Geometry check sheet. Reference: the model listing, model coordinates, mm. Round coordinates to 2 decimals unless told otherwise and drop trailing zeros. Write each loop counter-clockwise with the first axis right and the second up, starting at its lowest first coordinate (ties: lowest second). Pieces come first, ordered by that corner, then holes. Notation, with made-up numbers: M -1,70.25 L 22,70.25 A14 cw 22,79.25 Z; hole C 39,76 d11. An arc over 180 degrees is marked long. One line per item, written item: value. Start each with the question number.
1. Depth check by flat-ended pin: P1, Ø8, axis at x = 7, y = 14, coming from the -Z side; P2, Ø8, axis at y = 11.5, z = 778.5, coming from the +X side (3 decimals); P3, Ø5, axis at y = 6.5, z = 552.5, coming from the +X side; P4, Ø5, axis at x = 12, y = 7.5, coming from the -Z side. Enter the tip coordinate at first touch or a pass-through.
2. Scan lines: probe 1 along X at (y, z) = (18.5, 670.5) (3 decimals); probe 2 along Z at (x, y) = (1.75, 22.25). Record each from-to range of solid material in increasing order. Write a range as [from, to].
3. Section check C-C (y = 10.5). Record the boundary of the cut face in (x, z) (3 decimals).
4. Section check A-A (z = 879.5). Record the boundary of the cut face in (x, y) (3 decimals), and give its area (3 significant figures).
5. Section check B-B (x = 14). Record the boundary of the cut face in (y, z) (3 decimals).
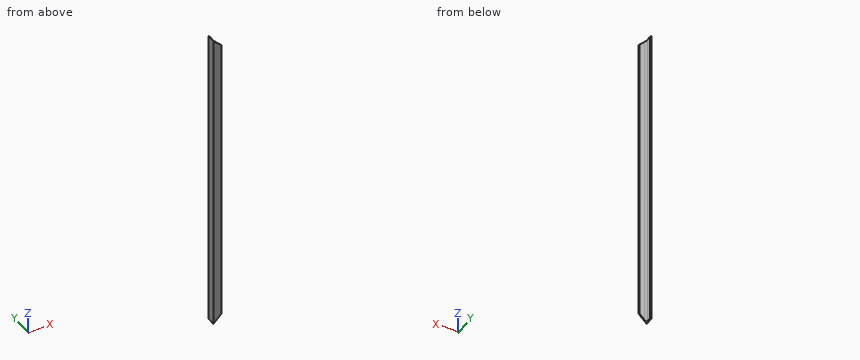
Autodesk Inventor part; units mm, degrees
ref_plane "Start Plane" through (0, 0, 0) normal (0, 0, 1) x (1, 0, 0)
ref_plane "End Plane" through (0, 0, 1000) normal (0, 0, 1) x (1, 0, 0)
ref_plane "Work Plane30" through (-0.0013, 12.7013, 0) normal (0.7071, -0.0001, -0.7071) x (-0.7071, 0.0002, -0.7071)
ref_plane "Start Plane" through (0, 0, 0) normal (0, 0, 1) x (1, 0, 0)
ref_plane "End Plane" through (0, 0, 1000) normal (0, 0, 1) x (1, 0, 0)
sketch "Sketch" plane through (0, 0, 0) normal (0, 0, 1) x (1, 0, 0)
  line L0 (25.4, 0) -> (0, 0)
  line L1 (0, 0) -> (0, 25.4)
  line L2 (0, 25.4) -> (1.651, 25.4)
  line L3 (3.175, 23.876) -> (3.175, 6.477)
  line L4 (6.477, 3.175) -> (23.876, 3.175)
  line L5 (25.4, 1.651) -> (25.4, 0)
  line L6 (0, -11.0414) -> (0, 31.5385) construction
  line L7 (-11.0414, 0) -> (31.5385, 0) construction
  arc A0 (3.175, 6.477) -> (6.477, 3.175) centre (6.477, 6.477) ccw
  arc A1 (3.175, 23.876) -> (1.651, 25.4) centre (1.651, 23.876) ccw
  arc A2 (25.4, 1.651) -> (23.876, 3.175) centre (23.876, 1.651) ccw
  line L8 (0, 40.0545) -> (0, -19.5574) construction
  line L9 (-19.5574, 0) -> (40.0545, 0) construction
  point P0 (3.175, 25.4)
  point P1 (3.175, 3.175)
  point P2 (25.4, 3.175)
  dimension "d0" = 25.4
  dimension "d1" = 25.4
  dimension "d2" = 3.175
  dimension "d3" = 3.175
  dimension "d10" = 0
  dimension "d11" = 0
  dimension "d14" = 3.302
  dimension "d15" = 1.524
extrude "Body" add sketch "Sketch" along normal up to surface (1000 mm away) from surface at 0
sketch "Sketch3" plane through (0, 0, 0) normal (0, 0, 1) x (1, 0, 0)
  line L0 (0, 0) -> (10, 0)
ref_plane "Work Plane3" through (0, 0, 0) normal (0, -1, 0) x (1, 0, 0)
ref_plane "Work Plane30" through (-0.0013, 12.7013, 0) normal (0.7071, -0.0001, -0.7071) x (-0.7071, 0.0002, -0.7071)
split "Split3" plane through (-0.0013, 12.7013, 0) removes the side toward (0.7071, -0.0001, -0.7071)
ref_plane "Work Plane31" through (-0.0013, 12.7013, 1000) normal (0.7071, -0.0001, 0.7071) x (0.7071, 0, -0.7071)
split "Split4" plane through (-0.0013, 12.7013, 1000) removes the side toward (0.7071, -0.0001, 0.7071)
sketch "Sketch13" plane through (6.477, 3.175, 993.5214) normal (0, 1, 0) x (1, 0, 0)
  circle A0 centre (9.7828, 273.923) radius 1.65
  circle A1 centre (9.7828, 466.623) radius 1.65
  circle A2 centre (9.7828, 519.423) radius 1.65
  circle A3 centre (9.7828, 712.123) radius 1.65
  circle A4 centre (9.7828, 764.923) radius 1.65
  circle A5 centre (9.7828, 957.623) radius 1.65
  ellipse E0 centre (-0.4433, 28.423) end of major axis (-0.4433, 26.773) minor radius 1.6494
  ellipse E1 centre (-0.2869, 221.123) end of major axis (-0.2869, 219.473) minor radius 1.6494
  point P0 (-6.477, 993.5214)
sketch "Sketch14" plane through (3.175, 6.477, 996.8234) normal (1, 0, 0) x (0, 0, -1)
  circle A0 centre (277.225, 10.0627) radius 1.65
  circle A1 centre (469.925, 10.0627) radius 1.65
  circle A2 centre (522.725, 10.0627) radius 1.65
  circle A3 centre (715.425, 10.0627) radius 1.65
  circle A4 centre (768.225, 10.0627) radius 1.65
  circle A5 centre (960.925, 10.0627) radius 1.65
  ellipse E0 centre (31.725, 9.675) end of major axis (30.075, 9.675) minor radius 1.6494
  ellipse E1 centre (224.425, 9.675) end of major axis (226.075, 9.675) minor radius 1.6494
  point P0 (996.8234, -6.477)
sketch "Sketch4" plane through (0, 0, 0) normal (0, -1, 0) x (1, 0, 0)
  line L0 (-3.582, 0) -> (21.4918, 0)
  line L1 (-3.582, 1000) -> (21.4918, 1000)
  dimension "d17" = 1000
equation "\"d0\" = G_H"
equation "\"d1\" = G_H"
equation "\"d2\" = G_T"
equation "\"d3\" = G_T"
equation "\"d14\" = G_IR"
equation "\"d15\" = G_ER"
equation "\"d4\" = G_L"
equation "\"G_H\" = 25.4"
equation "\"G_T\" = 3.175"
equation "\"G_ER\" = 1.524"
equation "\"G_IR\" = 3.302"
equation "\"G_L\" = 1000"
equation "\"ex\" = 0"
equation "\"G_OFFSET_START\" = 0"
equation "\"G_OFFSET_END\" = 0"
properties part number "AISC - L 1 x 1 x 1/8 - 39.37" material "Steel, Mild"
Result sheet:
1. P1: stops at z = 3
1. P2: stops at x = 3.175
1. P3: stops at x = 4.29
1. P4: passes through
2. probe 1: x = [0, 3.175]
2. probe 2: z = [1.75, 998.25]
3. outline: M 0,0.002 L 3.175,3.177 L 3.175,996.823 L 0,999.998 Z
4. outline: M 0,0 L 25.4,0 L 25.4,1.651 A1.524 ccw 23.876,3.175 L 6.477,3.175 A3.302 cw 3.175,6.477 L 3.175,23.876 A1.524 ccw 1.651,25.4 L 0,25.4 Z
4. area: 153 mm2
5. outline: M 0,14.003 L 3.175,14.003 L 3.175,985.997 L 0,985.997 Z
